Check sheet for the modelled part. Datum: model origin and axes. Units: mm. A direction names the side the tool comes from. Give positions to 0.01 mm unless a question says otherwise; leave off trailing zeros. Loops run counter-clockwise (first coordinate to the right, second up) from the corner with the lowest first, then second, coordinate; pieces in that order, holes last. Notation, with made-up numbers: (-17, 42.5) - (34, 42.5) arc R30 ccw to (34, 71.5) - close; hole circle Ø3 at (54.25, 78). An arc over 180 degrees is marked (long way). Answer in a Markdown table with one row per item. Add a question column.
(1) Thickness scan on L1, parallel to Z at x = 122.5, y = 115.5; L2, parallel to X at y = 25, z = 64.5; L3, parallel to Z at x = -48, y = 115. Record the ranges inside material, lowest first.
(2) Draft check along Y on faces 3 (the face through (-47.769, 62, 52)), 4 (the face through (36, -2.5, 52)), 5 (the face through (36, 0, 52)), 6 (the face through (123.3, 113.8, 27.5)). Enter one of: released by +Y, released by -Y, zero draft, split by the parting line, or undercut.
(3) Sectioned sample at B-B on z = 105. Enter the section's corners in (x, y), then the cut area to 3 significant figures.
(4) Sectioned sample at A-A on y = 61. Enter the section's corners in (x, z).
(5) Sectioned sample at C-C on x = 98.5. Enter the section's corners in (y, z), then the cut area to 4 significant figures.
(6) Set-up check for faces 1 (the face through (123.3, 113.8, 78.5)), 2 (the face through (122.231, 62, 54)): record each of +Z, -Z, +X, -X, +Y, -Y from which the full face is reachable in a straight line by a thin tool's end or side.
(7) Go/stop test with flat-tipped pins: P1, Ø4, axis at y = 115.5, z = 128.27, coming from the +X side; P2, Ø4, axis at y = 115.5, z = -22.73, coming from the -X side. Record where each tip stops, or that it passes through.
from build123d import *

# Parameters (mm, degrees)
SKETCH_238_W                                   = 170
SKETCH_238_H                                   = 167
BASE_FLANGE1_DEPTH                             = 2.5
EDGE_FLANGE1_STRIP_W                           = 13
EDGE_FLANGE1_STRIP_H                           = 2.5
EDGE_FLANGE1_STRIP_CUT_DEPTH                   = 167
EDGE_FLANGE1_DEPTH                             = 167
EDGE_FLANGE2_STRIP_W                           = 13
EDGE_FLANGE2_STRIP_H                           = 2.5
EDGE_FLANGE2_STRIP_CUT_DEPTH                   = 167
EDGE_FLANGE2_DEPTH                             = 167
CSK_FOR_M3_FLAT_HEAD_MACHINE_SCREW1_AT_2_COUNT = 2
CSK_FOR_M3_FLAT_HEAD_MACHINE_SCREW1_AT_2_PITCH = 50
CSK_FOR_M3_FLAT_HEAD_MACHINE_SCREW1_AT_3_COUNT = 2
CSK_FOR_M3_FLAT_HEAD_MACHINE_SCREW1_AT_3_PITCH = 101
CSK_FOR_M3_FLAT_HEAD_MACHINE_SCREW1_AT_4_COUNT = 2
CSK_FOR_M3_FLAT_HEAD_MACHINE_SCREW1_AT_4_PITCH = 151
CSK_FOR_M3_FLAT_HEAD_MACHINE_SCREW2_AT_2_COUNT = 2
CSK_FOR_M3_FLAT_HEAD_MACHINE_SCREW2_AT_2_PITCH = 50
CSK_FOR_M3_FLAT_HEAD_MACHINE_SCREW2_AT_3_COUNT = 2
CSK_FOR_M3_FLAT_HEAD_MACHINE_SCREW2_AT_3_PITCH = 101
CSK_FOR_M3_FLAT_HEAD_MACHINE_SCREW2_AT_4_COUNT = 2
CSK_FOR_M3_FLAT_HEAD_MACHINE_SCREW2_AT_4_PITCH = 151


# Sheet-metal steps are written as plain solids
with BuildPart() as part:
    # Sketch 238 → Base-Flange1 (new body)
    with BuildSketch(Plane(origin=(0, 0, 0), x_dir=(1, 0, 0), z_dir=(0, 1, 0))):
        with Locations((37.231404959, -52.766528926)):
            Rectangle(SKETCH_238_W, SKETCH_238_H)
    extrude(amount=-BASE_FLANGE1_DEPTH)

    # Edge-Flange1 strip (across the edge) → Edge-Flange1 strip cut (cut)
    with BuildSketch(Plane(origin=(-47.768595041, 0, -30.733471074), x_dir=(1, 0, 0), z_dir=(0, 0, 1))):
        with Locations((-5, -1.25)):
            Rectangle(EDGE_FLANGE1_STRIP_W, EDGE_FLANGE1_STRIP_H)
    extrude(amount=EDGE_FLANGE1_STRIP_CUT_DEPTH, mode=Mode.SUBTRACT)

    # Edge-Flange1 section (across the edge) → Edge-Flange1 (add)
    with BuildSketch(Plane(origin=(-47.768595041, 0, -30.733471074), x_dir=(1, 0, 0), z_dir=(0, 0, 1))):
        with BuildLine():
            Line((-2.5, 1.5), (-2.5, 120.5))
            Line((-2.5, 120.5), (0, 120.5))
            Line((0, 120.5), (0, 1.5))
            ThreePointArc((0, 1.5), (0.439339828, 0.439339828), (1.5, 0))
            Line((1.5, 0), (1.5, -2.5))
            ThreePointArc((1.5, -2.5), (-1.328427125, -1.328427125), (-2.5, 1.5))
        make_face()
    extrude(amount=EDGE_FLANGE1_DEPTH)

    # Edge-Flange2 strip (across the edge) → Edge-Flange2 strip cut (cut)
    with BuildSketch(Plane(origin=(122.231404959, 0, 136.266528926), x_dir=(-1, 0, 0), z_dir=(0, 0, -1))):
        with Locations((-5, -1.25)):
            Rectangle(EDGE_FLANGE2_STRIP_W, EDGE_FLANGE2_STRIP_H)
    extrude(amount=EDGE_FLANGE2_STRIP_CUT_DEPTH, mode=Mode.SUBTRACT)

    # Edge-Flange2 section (across the edge) → Edge-Flange2 (add)
    with BuildSketch(Plane(origin=(122.231404959, 0, 136.266528926), x_dir=(-1, 0, 0), z_dir=(0, 0, -1))):
        with BuildLine():
            Line((-2.5, 1.5), (-2.5, 120.5))
            Line((-2.5, 120.5), (0, 120.5))
            Line((0, 120.5), (0, 1.5))
            ThreePointArc((0, 1.5), (0.439339828, 0.439339828), (1.5, 0))
            Line((1.5, 0), (1.5, -2.5))
            ThreePointArc((1.5, -2.5), (-1.328427125, -1.328427125), (-2.5, 1.5))
        make_face()
    extrude(amount=EDGE_FLANGE2_DEPTH)

    # Sketch13 → CSK for M3 Flat Head Machine Screw1 (revolve, cut)
    with BuildSketch(Plane(origin=(-50.268595041, 115.5, 128.266528926), x_dir=(0, 0, 1), z_dir=(0, 1, 0))):
        Polygon((0, 0), (0, 2.5), (1.6, 2.5), (1.6, 1.55), (3.15, 0), align=None)
    csk_for_m3_flat_head_machine_screw1 = revolve(axis=Axis((-56.618595041, 115.5, 128.266528926), (1, 0, 0)), mode=Mode.SUBTRACT)

    # CSK for M3 Flat Head Machine Screw1 at 2: CSK for M3 Flat Head Machine Screw1 ×2
    with Locations(*[(0, 0, -i * CSK_FOR_M3_FLAT_HEAD_MACHINE_SCREW1_AT_2_PITCH) for i in range(1, CSK_FOR_M3_FLAT_HEAD_MACHINE_SCREW1_AT_2_COUNT)]):
        add(csk_for_m3_flat_head_machine_screw1, mode=Mode.SUBTRACT)

    # CSK for M3 Flat Head Machine Screw1 at 3: CSK for M3 Flat Head Machine Screw1 ×2
    with Locations(*[(0, 0, -i * CSK_FOR_M3_FLAT_HEAD_MACHINE_SCREW1_AT_3_PITCH) for i in range(1, CSK_FOR_M3_FLAT_HEAD_MACHINE_SCREW1_AT_3_COUNT)]):
        add(csk_for_m3_flat_head_machine_screw1, mode=Mode.SUBTRACT)

    # CSK for M3 Flat Head Machine Screw1 at 4: CSK for M3 Flat Head Machine Screw1 ×2
    with Locations(*[(0, 0, -i * CSK_FOR_M3_FLAT_HEAD_MACHINE_SCREW1_AT_4_PITCH) for i in range(1, CSK_FOR_M3_FLAT_HEAD_MACHINE_SCREW1_AT_4_COUNT)]):
        add(csk_for_m3_flat_head_machine_screw1, mode=Mode.SUBTRACT)

    # Sketch15 → CSK for M3 Flat Head Machine Screw2 (revolve, cut)
    with BuildSketch(Plane(origin=(124.731404959, 115.5, -22.733471074), x_dir=(0, 0, -1), z_dir=(0, 1, 0))):
        Polygon((0, 0), (0, 2.5), (1.6, 2.5), (1.6, 1.55), (3.15, 0), align=None)
    csk_for_m3_flat_head_machine_screw2 = revolve(axis=Axis((131.081404959, 115.5, -22.733471074), (-1, 0, 0)), mode=Mode.SUBTRACT)

    # CSK for M3 Flat Head Machine Screw2 at 2: CSK for M3 Flat Head Machine Screw2 ×2
    with Locations(*[(0, 0, i * CSK_FOR_M3_FLAT_HEAD_MACHINE_SCREW2_AT_2_PITCH) for i in range(1, CSK_FOR_M3_FLAT_HEAD_MACHINE_SCREW2_AT_2_COUNT)]):
        add(csk_for_m3_flat_head_machine_screw2, mode=Mode.SUBTRACT)

    # CSK for M3 Flat Head Machine Screw2 at 3: CSK for M3 Flat Head Machine Screw2 ×2
    with Locations(*[(0, 0, i * CSK_FOR_M3_FLAT_HEAD_MACHINE_SCREW2_AT_3_PITCH) for i in range(1, CSK_FOR_M3_FLAT_HEAD_MACHINE_SCREW2_AT_3_COUNT)]):
        add(csk_for_m3_flat_head_machine_screw2, mode=Mode.SUBTRACT)

    # CSK for M3 Flat Head Machine Screw2 at 4: CSK for M3 Flat Head Machine Screw2 ×2
    with Locations(*[(0, 0, i * CSK_FOR_M3_FLAT_HEAD_MACHINE_SCREW2_AT_4_PITCH) for i in range(1, CSK_FOR_M3_FLAT_HEAD_MACHINE_SCREW2_AT_4_COUNT)]):
        add(csk_for_m3_flat_head_machine_screw2, mode=Mode.SUBTRACT)


solid = part.part
Reply:
| question | item | result |
|---|---|---|
| 1 | L1 | -30.73 to -24.33, -21.13 to 25.67, 28.87 to 76.67, 79.87 to 126.67, 129.87 to 136.27 |
| 1 | L2 | -50.27 to -47.77, 122.23 to 124.73 |
| 1 | L3 | -30.73 to -24.25, -21.21 to 25.75, 28.79 to 76.75, 79.79 to 126.75, 129.79 to 136.27 |
| 2 | face 3 | zero draft |
| 2 | face 4 | released by -Y |
| 2 | face 5 | released by +Y |
| 2 | face 6 | undercut |
| 3 | outline | (-50.27, 1.5) arc R4 ccw to (-46.27, -2.5) - (120.73, -2.5) arc R4 ccw to (124.73, 1.5) - (124.73, 120.5) - (122.23, 120.5) - (122.23, 1.5) arc R1.5 cw to (120.73, 0) - (-46.27, 0) arc R1.5 cw to (-47.77, 1.5) - (-47.77, 120.5) - (-50.27, 120.5) - close |
| 3 | area | 1,030 mm^2 |
| 4 | outline | (-50.27, -30.73) - (-47.77, -30.73) - (-47.77, 136.27) - (-50.27, 136.27) - close; (122.23, -30.73) - (124.73, -30.73) - (124.73, 136.27) - (122.23, 136.27) - close |
| 5 | outline | (-2.5, -30.73) - (0, -30.73) - (0, 136.27) - (-2.5, 136.27) - close |
| 5 | area | 417.5 mm^2 |
| 6 | face 1 | +X |
| 6 | face 2 | +Z, -Z, +Y |
| 7 | P1 | x = 123.58 |
| 7 | P2 | x = -49.12 |
